from build123d import *

# Parameters (mm, degrees)
SKETCH2_R           = 43.044310864
BOSS_EXTRUDE1_DEPTH = 5
SKETCH3_R           = 3.589046815
BOSS_EXTRUDE2_DEPTH = 5
SKETCH4_R           = 13.044310864
BOSS_EXTRUDE3_DEPTH = 5


with BuildPart() as part:
    # Sketch2 → Boss-Extrude1 (new body)
    with BuildSketch(Plane.XY):
        Circle(SKETCH2_R)
    extrude(amount=BOSS_EXTRUDE1_DEPTH)

    # Sketch3 → Boss-Extrude2 (add)
    with BuildSketch(Plane.XY.offset(5)):
        with Locations((28.73518241, 0)):
            Circle(SKETCH3_R)
    extrude(amount=BOSS_EXTRUDE2_DEPTH)

    # Sketch4 → Boss-Extrude3 (add)
    with BuildSketch(Plane(origin=(0, 0, 0), x_dir=(-1, 0, 0), z_dir=(0, 0, -1))):
        Circle(SKETCH4_R)
    extrude(amount=BOSS_EXTRUDE3_DEPTH)


solid = part.part
Read the model definition and answer for the solid it produces. Units are mm, in the model's axes. A direction names the side the tool comes from. Give positions to 0.01 mm unless a question says otherwise; leave off trailing zeros. Write each loop counter-clockwise with the first axis right and the second up, starting at its lowest first coordinate (ties: lowest second). Pieces come first, ordered by that corner, then holes. Notation, with made-up numbers: (29, 62.25) -> (41, 62.25) arc R11 cw to (41, 77.25) -> close; hole circle Ø7 at (10, 41.5). An arc over 180 degrees is marked (long way). Answer as a JSON object with one key per item and string values. Group by question number.
1) Find section D-D (y = -31). Write down the section's boundary in (x, z), and give its area (3 significant figures).
2) Consider L1, parallel to Z at x = -4, y = -14; L2, parallel to Z at x = 31, y = 0; L3, parallel to Y at x = 14.5, z = 0.75. Determine where each line is inside the solid, lowest interval first. Write a range as from..to.
3) Each of these flat-tipped pins is pushed along its axis until it touches: P1, Ø3, axis at y = -17.5, z = 3.5, coming from the -X side; P2, Ø2, axis at y = -11, z = 1.5, coming from the -X side; P3, Ø3, axis at x = 3, y = 29, coming from the -Z side. Where does it stop, or does it pass through?
4) Find section C-C (x = -9.5). Write down the section's boundary in (y, z), and give its area (3 significant figures).
5) Find section A-A (x = 0). Write down the section's boundary in (y, z), and give its area (3 significant figures).
6) A tool of negligible diameter and unlimited length cuts with its end or side. For faces 1 (the cylindrical face through (25.15, 0.16, 7.46)), 2 (the flat face through (29, 0, 10)), 3 (the flat face through (9, 10, 0)), from which of +Z, -Z, +X, -X, +Y, -Y can it reach the whole face along a straight path? Write none if from no direction.
7) Find section B-B (y = 0). Write down the section's boundary in (x, z), and give its area (3 significant figures).
Values follow:
{
 "1": {"outline": "(-29.86, 0) -> (29.86, 0) -> (29.86, 5) -> (-29.86, 5) -> close", "area": "299 mm2"},
 "2": {"L1": "z = 0..5", "L2": "z = 0..10", "L3": "y = -40.53..40.53"},
 "3": {"P1": "stops at x = -39.96", "P2": "stops at x = -41.87", "P3": "stops at z = 0"},
 "4": {"outline": "(-41.98, 0) -> (-8.94, 0) -> (-8.94, -5) -> (8.94, -5) -> (8.94, 0) -> (41.98, 0) -> (41.98, 5) -> (-41.98, 5) -> close", "area": "509 mm2"},
 "5": {"outline": "(-43.04, 0) -> (-13.04, 0) -> (-13.04, -5) -> (13.04, -5) -> (13.04, 0) -> (43.04, 0) -> (43.04, 5) -> (-43.04, 5) -> close", "area": "561 mm2"},
 "6": {"face 1": "+Z", "face 2": "+Z, +X, -X, +Y, -Y", "face 3": "-Z"},
 "7": {"outline": "(-43.04, 0) -> (-13.04, 0) -> (-13.04, -5) -> (13.04, -5) -> (13.04, 0) -> (43.04, 0) -> (43.04, 5) -> (32.32, 5) -> (32.32, 10) -> (25.15, 10) -> (25.15, 5) -> (-43.04, 5) -> close", "area": "597 mm2"}
}
